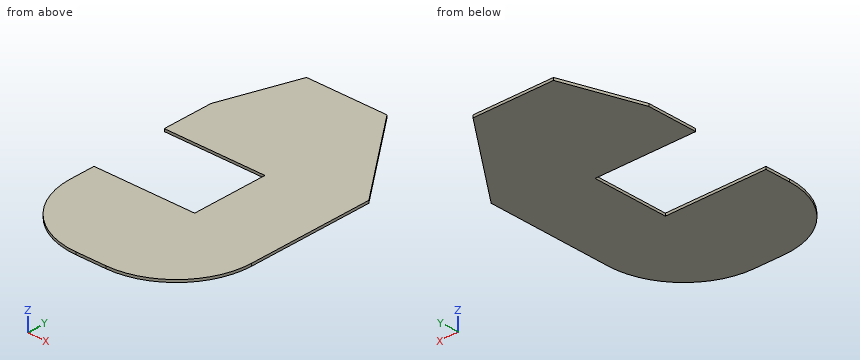
from build123d import *

# Parameters (mm, degrees)
F0_W     = 360
F0_H     = 600
F1_DEPTH = 5
F2_W     = 200
F2_H     = 150
F3_DEPTH = 25
F4_R     = 150
F5_SIZE2 = 50
F5_SIZE  = 150
F6_SIZE2 = 200
F6_SIZE  = 150
F7_R     = 150


with BuildPart() as f1:
    # F0 (on Top) → F1 (new body)
    with BuildSketch(Plane.XY):
        with Locations((180, 300)):
            Rectangle(F0_W, F0_H)
    extrude(amount=F1_DEPTH)

    # F2 (on face) → F3 (cut)
    with BuildSketch(Plane.XY.offset(5)):
        with Locations((100, 275)):
            Rectangle(F2_W, F2_H)
    extrude(amount=-F3_DEPTH, mode=Mode.SUBTRACT)

    # F4
    f4_edges = [f1.edges().sort_by_distance(p)[0] for p in [
        (0, 0, 2.5),
    ]]
    fillet(f4_edges, radius=F4_R)

    # F5
    f5_edges = [f1.edges().sort_by_distance(p)[0] for p in [
        (0, 600, 2.5),
    ]]
    f5_side = f1.faces().sort_by_distance((0, 475, 2.5))[0]
    chamfer(f5_edges, length=F5_SIZE, length2=F5_SIZE2, reference=f5_side)

    # F6
    f6_edges = [f1.edges().sort_by_distance(p)[0] for p in [
        (360, 600, 2.5),
    ]]
    f6_side = f1.faces().sort_by_distance((205, 600, 2.5))[0]
    chamfer(f6_edges, length=F6_SIZE, length2=F6_SIZE2, reference=f6_side)

    # F7
    f7_edges = [f1.edges().sort_by_distance(p)[0] for p in [
        (360, 0, 2.5),
    ]]
    fillet(f7_edges, radius=F7_R)


solid = f1.part
Work out the finished part from the listing and answer in its coordinate system (mm). Round coordinates to 2 decimals unless told otherwise and drop trailing zeros. Order: outer loops, then holes, each group sorted by start corner. A loop starts at its lowest first (then second) coordinate and runs counter-clockwise, first axis right, second up. Notation, with made-up numbers: M 19.5,1.5 L 76.5,1.5 A16 cw 76.5,24.5 Z; hole C -6,-22 d3. An arc over 180 degrees is marked long. Put each result on its own line as item: value. Start each with the question number.
Q1. Straight lines are drawn through the part: L1, parallel to Y at x = 184, z = 2.65; L2, parallel to Y at x = 86, z = 3.6; L3, parallel to X at y = 251, z = 4.55. For each, find the intervals that lie inside material, in ascending order. Write a range as [from, to].
Q2. Section C-C, the plane y = 427 is taken. Write down the section's boundary in (x, z), and give its area (3 significant figures).
Q3. A flat-ended cylindrical pin translates along its axis: pin 1 (1.5 mm diameter, centred on y = 266.5, z = 2.5, fed in from -X). Find the tip coordinate at first contact, or state that the pin passes through.
Q4. Section B-B, the plane z = 1.25 is taken. Write down the section's boundary in (x, y), and give its area (3 significant figures).
Q5. Section A-A, the plane x = 87 is taken. Write down the section's boundary in (y, z).
Q6. Section D-D, the plane x = 237 is taken. Write down the section's boundary in (y, z), and give its area (3 significant figures).
Findings below:
1. L1: y = [0, 200], [350, 600]
1. L2: y = [14.34, 200], [350, 600]
1. L3: x = [200, 360]
2. outline: M 0,0 L 339.75,0 L 339.75,5 L 0,5 Z
2. area: 1,700 mm^2
3. pin 1: stops at x = 200
4. outline: M 0,150 A150 ccw 150,0 L 210,0 A150 ccw 360,150 L 360,400 L 210,600 L 50,600 L 0,450 L 0,350 L 200,350 L 200,200 L 0,200 Z
4. area: 158,000 mm^2
5. outline: M 13.87,0 L 200,0 L 200,5 L 13.87,5 Z; M 350,0 L 600,0 L 600,5 L 350,5 Z
6. outline: M 2.45,0 L 564,0 L 564,5 L 2.45,5 Z
6. area: 2,810 mm^2
